from build123d import *

# Parameters (mm, degrees)
BOSS_EXTRUDE1_DEPTH = 4
SKETCH2_R           = 3.769998475
BOSS_EXTRUDE3_DEPTH = 6
SKETCH3_R           = 5.590277894
BOSS_EXTRUDE4_DEPTH = 1
DOME2_FACE_RADIUS   = 5.590277894
DOME2_HEIGHT        = 10


with BuildPart() as part:
    # Sketch1 → Boss-Extrude1 (new body)
    with BuildSketch(Plane(origin=(0, 0, 0), x_dir=(0, 0, -1), z_dir=(1, 0, 0))):
        with BuildLine():
            Line((19.618899977, 26.910578021), (30.093333643, 27.382443553))
            ThreePointArc((30.093333643, 27.382443553), (33.830584617, 25.946191816), (35.315810998, 22.228132309))
            Line((35.315810998, 22.228132309), (35.134279712, 16.536003005))
            ThreePointArc((35.134279712, 16.536003005), (33.751052045, 13.24033598), (30.52098964, 11.710160572))
            Line((30.52098964, 11.710160572), (19.560243471, 10.86550754))
            ThreePointArc((19.560243471, 10.86550754), (15.990018512, 12.15019262), (14.579969631, 15.672788846))
            Line((14.579969631, 15.672788846), (14.848236342, 22.1234032))
            ThreePointArc((14.848236342, 22.1234032), (16.302281821, 25.445064899), (19.618899977, 26.910578021))
        make_face()
    extrude(amount=BOSS_EXTRUDE1_DEPTH)

    # Sketch2 → Boss-Extrude3 (add)
    with BuildSketch(Plane(origin=(4, 0, 0), x_dir=(0, 0, -1), z_dir=(1, 0, 0))):
        with Locations(Location((22.478500698, 14.418661265, 0), (0, 0, 246.075553506))):
            Circle(SKETCH2_R)
    extrude(amount=BOSS_EXTRUDE3_DEPTH)

    # Sketch3 → Boss-Extrude4 (add)
    with BuildSketch(Plane(origin=(10, 0, 0), x_dir=(0, 0, -1), z_dir=(1, 0, 0))):
        with Locations((22.920717482, 14.60121679)):
            Circle(SKETCH3_R)
    extrude(amount=BOSS_EXTRUDE4_DEPTH)

    # Dome2: a dome of height H over a round flat face of radius A is a cap of a sphere of radius (A * A + H * H) / (2 * H)
    dome2_r = (DOME2_FACE_RADIUS * DOME2_FACE_RADIUS + DOME2_HEIGHT * DOME2_HEIGHT) / (2 * DOME2_HEIGHT)
    dome2_base = Plane((11, 14.60121679, -22.920717482), z_dir=(1, 0, 0))
    with Locations(dome2_base.offset(DOME2_HEIGHT - dome2_r)):
        dome2_ball = Sphere(dome2_r, mode=Mode.PRIVATE)
    add(split(dome2_ball, bisect_by=dome2_base, keep=Keep.TOP, mode=Mode.PRIVATE))


solid = part.part
Design review of the part built by this model. Coordinates are the model's own, in mm. A direction names the side the tool comes from. Give positions to 0.01 mm unless a question says otherwise; leave off trailing zeros. Order: outer loops, then holes, each group sorted by start corner. A loop starts at its lowest first (then second) coordinate and runs counter-clockwise, first axis right, second up.
1. Add section B-B, the plane x = 3.5. State the section outline as (y, z) points.
Solution:
outline: (10.87, -19.56) - (11.71, -30.52) arc R5 ccw to (16.54, -35.13) - (22.23, -35.32) arc R5 ccw to (27.38, -30.09) - (26.91, -19.62) arc R5 ccw to (22.12, -14.85) - (15.67, -14.58) arc R4.63 ccw to start
2. Tool access review of faces 1 (the flat face through (1.972, 11.294, -25.117)), 2 (the flat face through (10, 15, -27)), 3 (the cylindrical face through (1.97, 13.28, -33.79)): name each direction out of +Z, -Z, +X, -X, +Y, -Y from which nothing blocks a thin tool from reaching the whole face with its end or side.
Solution:
face 1: -Z, -X, -Y
face 2: none
face 3: -Z, +X, -X, -Y
3. Add section D-D, the plane z = -23.5. State the section outline as (x, y) points, then the cut area to 3 significant figures.
Solution:
outline: (0, 11.17) - (4, 11.17) - (4, 10.79) - (10, 10.79) - (10, 9.04) - (11, 9.04) arc R6.54 ccw (long way) to (11, 20.16) - (10, 20.16) - (10, 18.05) - (4, 18.05) - (4, 27.09) - (0, 27.09) - close
area: 228 mm2
4. Add section C-C, the plane y = 13.25. State the section outline as (x, z) points.
Solution:
outline: (0, -33.76) - (4, -33.76) - (4, -26.06) - (10, -26.06) - (10, -28.35) - (11, -28.35) arc R6.42 ccw (long way) to (11, -17.5) - (10, -17.5) - (10, -18.89) - (4, -18.89) - (4, -15.15) - (0, -15.15) - close
5. Add section A-A, the plane z = -18. State the section outline as (x, y) points, then the cut area to 3 significant figures.
Solution:
outline: (0, 11.01) - (4, 11.01) - (4, 26.56) - (0, 26.56) - close; (10, 11.95) - (11, 11.95) arc R4.34 ccw (long way) to (11, 17.25) - (10, 17.25) - close
area: 123 mm2
6. For pin 1 Ø4 at (y, z) = (18.5, -27) entering from +X; pin 2 Ø6 at (y, z) = (16, -32) entering from -X; pin 3 Ø6 at (y, z) = (21, -20) entering from +X; pin 4 Ø6 at (x, z) = (11, -23.5) entering from -Y, all flat-tipped, find the tip position at first contact; note any pin that passes through.
Solution:
pin 1: stops at x = 19.9
pin 2: stops at x = 0
pin 3: stops at x = 19.61
pin 4: stops at y = 8.06
7. To check wall thickness, follow L1, parallel to X at y = 24, z = -22.25; L2, parallel to X at y = 13.5, z = -18.75; L3, parallel to X at y = 10.25, z = -19.75. State the ranges of each line that lie inside material, in increasing order.
Solution:
L1: x = 0 to 4
L2: x = 0 to 4, 10 to 19.38
L3: x = 10 to 18.19
